Could you check a few things on this drawing? It's one solid part, dimensions in mm from its lowest x, y, z. A direction names the side the tool comes from. Round coordinates to 2 decimals unless told otherwise and drop trailing zeros. Write each loop counter-clockwise with the first axis right and the second up, starting at its lowest first coordinate (ties: lowest second). Pieces come first, ordered by that corner, then holes. Notation, with made-up numbers: (47.5, 0) -> (91.5, 0) arc R20 ccw to (91.5, 14) -> close; hole circle Ø1 at (-20.5, 38). An arc over 180 degrees is marked (long way). Answer in a Markdown table with one row per item.
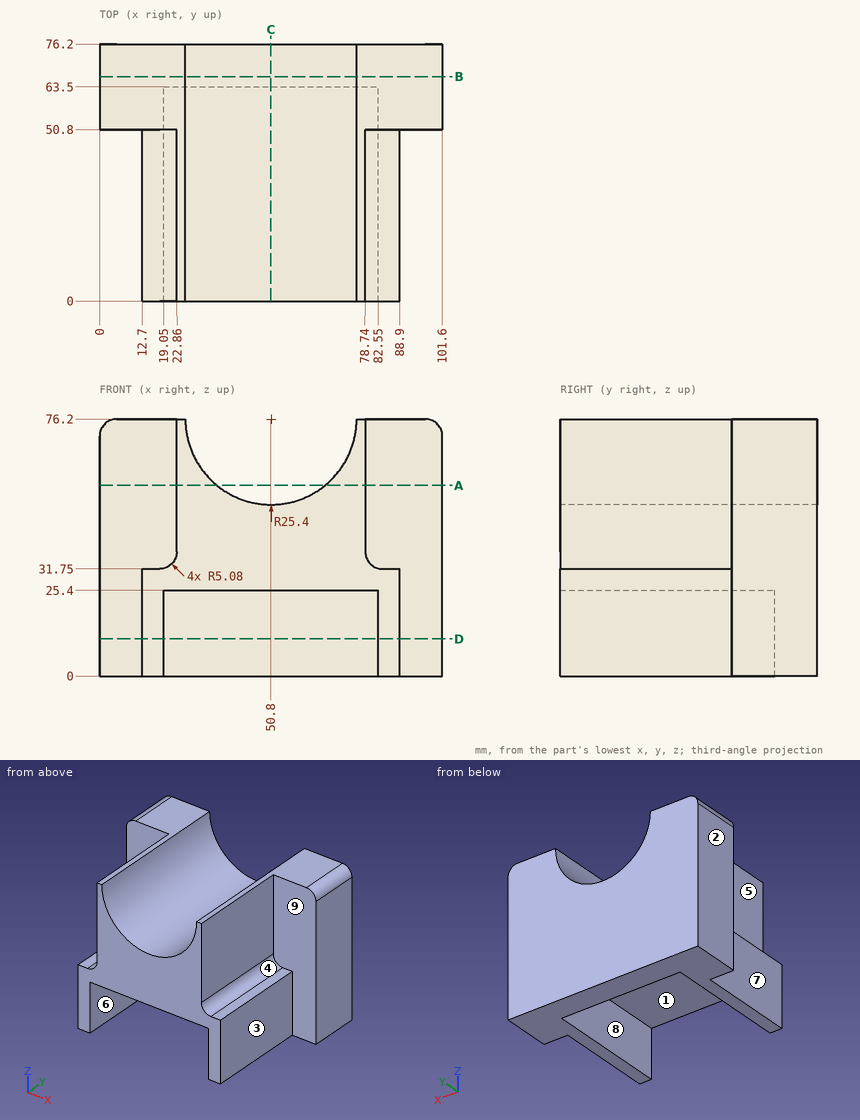
1) Which directions (+Z, -Z, +X, -X, +Y, -Y) give clear straight access to the entire face, cutting with the end or side of a thin tool? Please do the marked faces 1, 2, 3, 4 and 5.
Response:
| item | result |
|---|---|
| face 1 | -Z, -Y |
| face 2 | +Z, -Z, -X, +Y, -Y |
| face 3 | +Z, -Z, +X, -Y |
| face 4 | +Z, +X, -Y |
| face 5 | +Z, -X, -Y |
2) I want a section at A-A, the plane z = 56.5. List the corners of the cut face in (x, y) for me, and give its area (3 significant figures).
Response:
| item | result |
|---|---|
| outline | (0, 50.8) -> (22.86, 50.8) -> (22.86, 0) -> (34.77, 0) -> (34.77, 76.2) -> (0, 76.2) -> close; (66.83, 0) -> (78.74, 0) -> (78.74, 50.8) -> (101.6, 50.8) -> (101.6, 76.2) -> (66.83, 76.2) -> close |
| area | 2,980 mm^2 |
3) For pin 1 (1.5 mm diameter, centred on x = 86.5, y = 36.5, fed in from +Z); pin 2 (16 mm diameter, centred on y = 22.5, z = 11, fed in from -X); pin 3 (25 mm diameter, centred on x = 6.5, z = 46, fed in from -Y), each with a flat end and sliding along its axis, tell me the tip position at first contact or that it passes through.
Response:
| item | result |
|---|---|
| pin 1 | stops at z = 31.75 |
| pin 2 | stops at x = 12.7 |
| pin 3 | stops at y = 50.8 |
4) I want a section at B-B, the plane y = 66.5. List the corners of the cut face in (x, z) for me, and give its area (3 significant figures).
Response:
| item | result |
|---|---|
| outline | (0, 0) -> (101.6, 0) -> (101.6, 71.12) arc R5.08 ccw to (96.52, 76.2) -> (76.2, 76.2) arc R25.4 cw to (25.4, 76.2) -> (5.08, 76.2) arc R5.08 ccw to (0, 71.12) -> close |
| area | 6,720 mm^2 |
5) I want a section at D-D, the plane z = 11. List the corners of the cut face in (x, y) for me.
Response:
| item | result |
|---|---|
| outline | (0, 50.8) -> (12.7, 50.8) -> (12.7, 0) -> (19.05, 0) -> (19.05, 63.5) -> (82.55, 63.5) -> (82.55, 0) -> (88.9, 0) -> (88.9, 50.8) -> (101.6, 50.8) -> (101.6, 76.2) -> (0, 76.2) -> close |
6) I need wall thicknesses on line 1 (X direction, y = 5, z = 16); line 2 (Z direction, x = 77.5, y = 24.5); line 3 (X direction, y = 46, z = 47). Which ranges of each line are inside material? Lowest first, please. Write a range as [from, to].
Response:
| item | result |
|---|---|
| line 1 | x = [12.7, 19.05], [82.55, 88.9] |
| line 2 | z = [25.4, 76.2] |
| line 3 | x = [22.86, 78.74] |
7) We'd pull the mould along X, two halves only. Please class the marked faces 6, 7, 8 and 9: +X half, -X half, draft (parallel to the pull), parting line (faces both ways), or undercut.
Response:
| item | result |
|---|---|
| face 6 | undercut |
| face 7 | -X half |
| face 8 | undercut |
| face 9 | draft |
8) I want a section at C-C, the plane x = 50.8. List the corners of the cut face in (y, z) for me, and give its area (3 significant figures).
Response:
| item | result |
|---|---|
| outline | (0, 25.4) -> (63.5, 25.4) -> (63.5, 0) -> (76.2, 0) -> (76.2, 50.8) -> (0, 50.8) -> close |
| area | 2,260 mm^2 |
